Solid Edge part; units mm, degrees
sketch "Sketch1" plane through (0, 0, 0) normal (0, -1, 0) x (1, 0, 0)
  line L0 (12, 15) -> (-12, 15)
  line L1 (-12, 15) -> (-12, -15)
  line L2 (-12, -15) -> (12, -15)
  line L3 (12, -15) -> (110, -25)
  line L4 (110, 0) -> (110, -25)
  line L5 (110, 0) -> (110, 25)
  line L6 (12, 15) -> (110, 25)
extrude "Protrusion1" add sketch "Sketch1" against normal blind 10
sketch "Sketch2" plane through (0, 5, 15) normal (0, 0, 1) x (-1, 0, 0)
  line L0 (12, 20) -> (12, -5)
  line L1 (12, -5) -> (-12, -5)
  line L2 (-12, -5) -> (-12, 20)
  arc A0 (-12, 20) -> (12, 20) centre (0, 20) cw
extrude "ExtrudedProtrusion_6" add sketch "Sketch2" against normal blind 9
sketch "Sketch3" plane through (0, 5, -15) normal (0, 0, -1) x (1, 0, 0)
  line L0 (12, 20) -> (12, -5)
  line L1 (12, -5) -> (-12, -5)
  line L2 (-12, -5) -> (-12, 20)
  arc A0 (-12, 20) -> (12, 20) centre (0, 20) cw
extrude "ExtrudedProtrusion_7" add sketch "Sketch3" against normal blind 9
sketch "Sketch4" plane through (0, -8.5, -15) normal (0, 0, -1) x (1, 0, 0)
  circle A0 centre (0, 6.5) radius 6
extrude "Cutout1" cut sketch "Sketch4" against normal through all
sketch "Sketch5" plane through (49, 0, 0) normal (0, -1, 0) x (0.9948, 0, -0.1015)
  circle A0 centre (60.6849, 6.1923) radius 25
extrude "ExtrudedProtrusion_11" add sketch "Sketch5" along normal blind 20 and the other way blind 30
sketch "Sketch6" plane through (110, -20, 0) normal (0, -1, 0) x (1, 0, 0)
  circle A0 centre (0, 0) radius 15
extrude "Cutout2" cut sketch "Sketch6" against normal through all
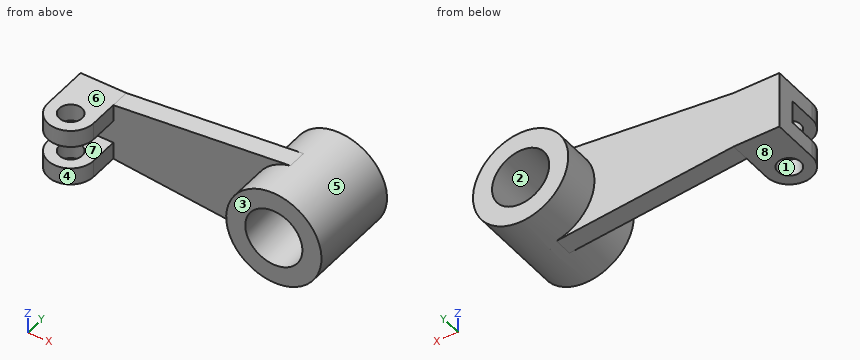
Geometry check sheet. Reference: the model listing, model coordinates, mm. Face numbers are marked on the shaded views. A direction names the side the tool comes from. Give positions to 0.01 mm unless a question says otherwise; leave off trailing zeros. Loops run counter-clockwise (first coordinate to the right, second up) from the corner with the lowest first, then second, coordinate; pieces in that order, holes last. Notation, with made-up numbers: (52, 79.5) - (102, 79.5) arc R14 ccw to (102, 96.5) - close; hole circle Ø5 at (-32.75, 72). An arc over 180 degrees is marked (long way). Use CSV: the item, a comma, the result in double quotes. Start each with the question number.
Q1. Section check D-D, the plane x = 122.5. Record the cut outline in (y, z), and give its area (3 significant figures).
Q2. Go/stop test with flat-tipped pins: pin 1 Ø25 at (x, z) = (119.5, -7.5) entering from -Y; pin 2 Ø10 at (y, z) = (-6, 6.5) entering from +X (3 decimals); pin 3 Ø4 at (x, y) = (65.5, 5) entering from +Z; pin 4 Ø12 at (y, z) = (-4, -17.5) entering from -X. Record where each tip stops, or that it passes through.
Q3. Section check C-C, the plane x = 0. Record the cut outline in (y, z), and give its area (3 significant figures).
Q4. Release check for a two-part mould opening along Y. For the marked faces 1, 2 and 3 record: +Y half, -Y half, draft (parallel to the pull), parting line (faces both ways), or undercut.
Q5. Section check B-B, the plane z = 0. Record the cut outline in (x, y), and give its area (3 significant figures).
Q6. Access from +Z, -Z, +X, -X, +Y, -Y to the whole of each face (thin tool, end or side, straight path). Record for the marked faces 4, 5, 6, 7 and 8.
Q7. Scan lines: probe 1 along Y at (x, z) = (0, -13); probe 2 along Z at (x, y) = (110, -4.5); probe 3 along Y at (x, z) = (19.5, -8). Record each from-to range of solid material in increasing order. Write a range as from..to.
Findings below:
1,outline,"(-20, -21.65) - (30, -21.65) - (30, -8.29) - (-20, -8.29) - close; (-20, 8.29) - (30, 8.29) - (30, 21.65) - (-20, 21.65) - close"
1,area,"1,340 mm^2"
2,pin 1,"stops at y = -20"
2,pin 2,"stops at x = 134.955"
2,pin 3,"stops at z = 20.66"
2,pin 4,"stops at x = -12"
3,outline,"(-27, -15) - (-21, -15) - (-21, -6) - (-27, -6) - close; (-27, 6) - (-21, 6) - (-21, 15) - (-27, 15) - close; (-9, -15) - (10, -15) - (10, 15) - (-9, 15) - (-9, 6) - (0, 6) - (0, -6) - (-9, -6) - close"
3,area,"570 mm^2"
4,face 1,"undercut"
4,face 2,"draft"
4,face 3,"-Y half"
5,outline,"(-12, 0) - (85, 0) - (85, -20) - (95, -20) - (95, 30) - (85, 30) - (85, 10) - (-12, 10) - close; (125, -20) - (135, -20) - (135, 30) - (125, 30) - close"
5,area,"1,970 mm^2"
6,face 4,"+Z, -Z, -Y"
6,face 5,"none"
6,face 6,"+Z, -X, +Y, -Y"
6,face 7,"-X, -Y"
6,face 8,"-Z, -X, +Y, -Y"
7,probe 1,"y = -27..-21, -9..10"
7,probe 2,"z = -25..-15, 15..25"
7,probe 3,"y = 0..10"
